Drawing for the job (mm, zero at the part's lowest x, y, z). A direction names the side the tool comes from. Round coordinates to 2 decimals unless told otherwise and drop trailing zeros. Write each loop counter-clockwise with the first axis right and the second up, starting at its lowest first coordinate (ties: lowest second). Pieces come first, ordered by that corner, then holes. Notation, with made-up numbers: (57, 10) - (115, 10) arc R23 cw to (115, 39) - close; hole circle Ø5 at (5, -37). An arc over 180 degrees is marked (long way). One line per question, with ' | ' between items.
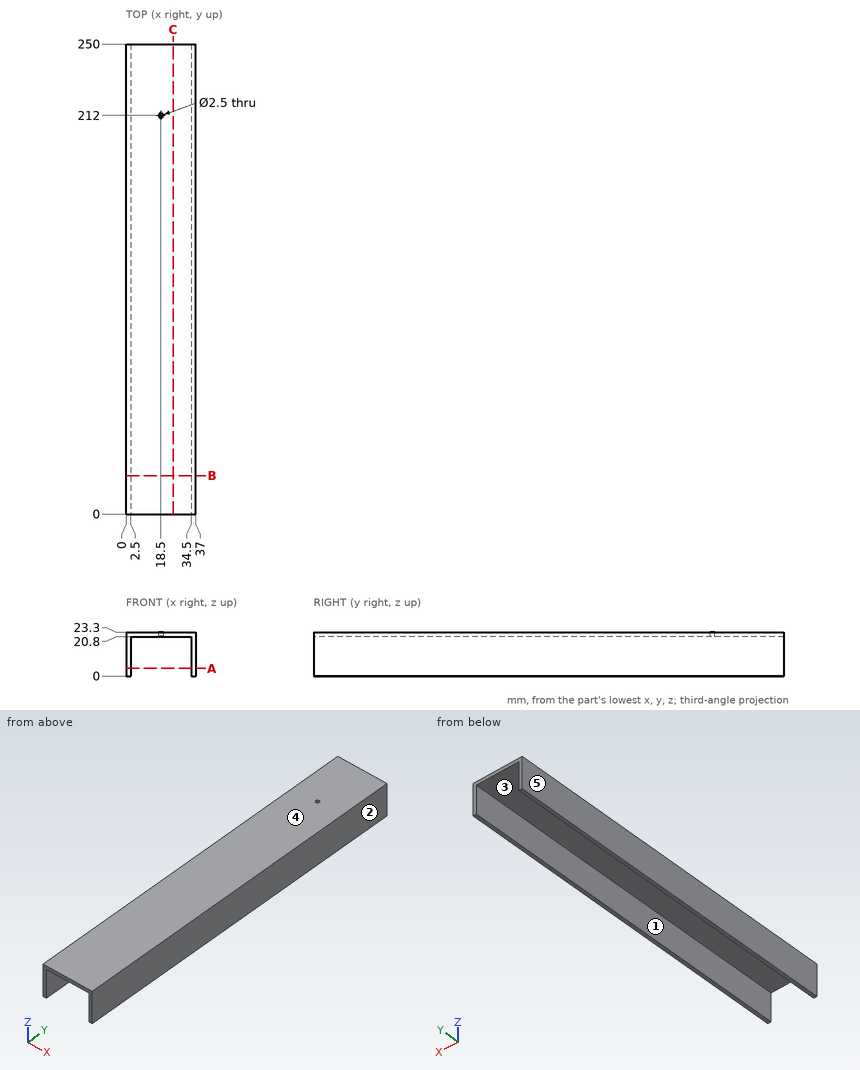
Q1. Pull direction X, two halves, no side cores. Call the marked faces 3, 4 and 5: +X half, -X half, draft (parallel to the pull), parting line (faces both ways), or undercut.
Found:
face 3: undercut | face 4: draft | face 5: -X half
Q2. Saw through at A-A, the plane z = 4. List the corners of the cut face in (x, y).
Found:
outline: (0, 0) - (2.5, 0) - (2.5, 250) - (0, 250) - close; (34.5, 0) - (37, 0) - (37, 250) - (34.5, 250) - close
Q3. Drop flat-ended pins along their axis: pin 1 (9.5 mm diameter, centred on x = 22, y = 66, fed in from -Z); pin 2 (6 mm diameter, centred on y = 145.5, z = 13.5, fed in from -X). Give the stop position or say it passes through.
Found:
pin 1: z = 20.8 | pin 2: x = 0
Q4. Which spindle directions (+Z, -Z, +X, -X, +Y, -Y) get a long thin tool onto all of the face, cutting with end or side? Do the marked faces 1 and 2. Say none if no direction does.
Found:
face 1: -Z, +Y, -Y | face 2: +Z, -Z, +X, +Y, -Y
Q5. Saw through at B-B, the plane y = 20.5. List the corners of the cut face in (x, z), then the cut area to 4 significant figures.
Found:
outline: (0, 0) - (2.5, 0) - (2.5, 20.8) - (34.5, 20.8) - (34.5, 0) - (37, 0) - (37, 23.3) - (0, 23.3) - close | area: 196.5 mm^2
Q6. Drill centre lines: L1, parallel to X at y = 212, z = 21.75; L2, parallel to X at y = 118, z = 17.25; L3, parallel to Y at x = 18.5, z = 22.4. Where is each one in solid material? Low to high. Write a range as from..to.
Found:
L1: 0..17.25, 19.75..37 | L2: 0..2.5, 34.5..37 | L3: 0..210.75, 213.25..250
Q7. Saw through at C-C, the plane x = 25. List the corners of the cut face in (y, z), then the cut area to 3 significant figures.
Found:
outline: (0, 20.8) - (250, 20.8) - (250, 23.3) - (0, 23.3) - close | area: 625 mm^2
